Geometry check sheet. Reference: the model listing, model coordinates, mm. A direction names the side the tool comes from. Coordinates: 2 decimals unless noted, no trailing zeros. Write each loop counter-clockwise with the first axis right and the second up, starting at its lowest first coordinate (ties: lowest second). Pieces come first, ordered by that corner, then holes. Notation, with made-up numbers: (-1.75, 63) -> (14.25, 63) arc R9 cw to (14.25, 67) -> close; hole circle Ø10 at (49, 89.25). An arc over 180 degrees is marked (long way). Answer in a Markdown table with one row per item. Add a question column.
Q1. Tool access check on faces 4 (the face through (-65, 60, -62)), 5 (the face through (-173.206, 54.768, -26.385)). Record the directions out of +Z, -Z, +X, -X, +Y, -Y that give a thin tool (end or side, any length) a straight path to the whole face; none if there is none.
Q2. Thickness scan on line 1 (X direction, y = 57.5, z = -85); line 2 (Y direction, x = -34, z = -34.5); line 3 (Y direction, x = 166.5, z = 21). Record the ranges inside material, lowest first.
Q3. Section check D-D, the plane z = 17.5. Record the boundary of the cut face in (x, y), and give its area (3 significant figures).
Q4. Section check A-A, the plane x = -44. Record the boundary of the cut face in (y, z).
Q5. Gauge pin test, flat ends, axial feed: P1, Ø3, axis at x = -179, z = 34.5, coming from the +Y side; P2, Ø4, axis at x = -185.5, z = -23, coming from the +Y side. Record the tip position at first contact, or that the pin passes through.
Q6. Release check for a two-part mould opening along Z. For faces 1 (the face through (-35, 53.5, -24)), 2 (the face through (-9, 30, -108.456)), 3 (the face through (-255.515, 30, -22)) record: pulls with the +Z half, pulls with the -Z half, needs draft (parallel to the pull), parting line crosses it, or undercut.
Q7. Section check B-B, the plane z = 37. Record the boundary of the cut face in (x, y), and give its area (3 significant figures).
Q8. Section check C-C, the plane x = 44. Record the boundary of the cut face in (y, z), and give its area (3 significant figures).
```python
from build123d import *

# Parameters (mm, degrees)
SKETCH1_W           = 500
SKETCH1_H           = 170
BOSS_EXTRUDE1_DEPTH = 60
SKETCH3_R           = 67.5
CUT_EXTRUDE1_DEPTH  = 4
SKETCH4_R           = 25
SKETCH4_R_2         = 22.5
CUT_EXTRUDE2_DEPTH  = 2.5


with BuildPart() as part:
    # Sketch1 → Boss-Extrude1 (new body)
    with BuildSketch(Plane(origin=(0, 0, 0), x_dir=(1, 0, 0), z_dir=(0, 1, 0))):
        with Locations((-5.514705882, 23.455882353)):
            Rectangle(SKETCH1_W, SKETCH1_H)
    extrude(amount=BOSS_EXTRUDE1_DEPTH)

    # Sketch3 → Cut-Extrude1 (cut)
    with BuildSketch(Plane(origin=(0, 60, 0), x_dir=(1, 0, 0), z_dir=(0, 1, 0))):
        with Locations(Location((-5.514705882, 26.094123359, 0), (0, 0, 270))):
            Circle(SKETCH3_R)
        with Locations(Location((154.485294118, 26.094123359, 0), (0, 0, 270))):
            Circle(SKETCH3_R)
        with Locations(Location((-165.514705882, 26.094123359, 0), (0, 0, 270))):
            Circle(SKETCH3_R)
    extrude(amount=-CUT_EXTRUDE1_DEPTH, mode=Mode.SUBTRACT)

    # Sketch4 → Cut-Extrude2 (cut)
    with BuildSketch(Plane(origin=(0, 56, 0), x_dir=(1, 0, 0), z_dir=(0, 1, 0))):
        with Locations(Location((-135.514705882, 23.455882353, 0), (0, 0, 270))):
            Circle(SKETCH4_R)
        with Locations(Location((-195.514705882, 23.455882353, 0), (0, 0, 270))):
            Circle(SKETCH4_R_2)
        with Locations(Location((-35.514705882, 23.455882353, 0), (0, 0, 270))):
            Circle(SKETCH4_R_2)
        with Locations(Location((24.485294118, 23.455882353, 0), (0, 0, 270))):
            Circle(SKETCH4_R)
        with Locations(Location((124.485294118, 23.455882353, 0), (0, 0, 270))):
            Circle(SKETCH4_R_2)
        with Locations(Location((184.485294118, 23.455882353, 0), (0, 0, 270))):
            Circle(SKETCH4_R)
    extrude(amount=-CUT_EXTRUDE2_DEPTH, mode=Mode.SUBTRACT)


solid = part.part
```
Calculated:
| question | item | result |
|---|---|---|
| 1 | face 4 | +Z, -Z, +X, -X, +Y |
| 1 | face 5 | +Y |
| 2 | line 1 | x = -255.51 to -198.47, -132.55 to -38.47, 27.45 to 121.53, 187.45 to 244.49 |
| 2 | line 2 | y = 0 to 53.5 |
| 2 | line 3 | y = 0 to 56 |
| 3 | outline | (-255.51, 0) -> (244.49, 0) -> (244.49, 60) -> (206.02, 60) -> (206.02, 56) -> (102.95, 56) -> (102.95, 60) -> (46.02, 60) -> (46.02, 56) -> (-57.05, 56) -> (-57.05, 60) -> (-113.98, 60) -> (-113.98, 56) -> (-217.05, 56) -> (-217.05, 60) -> (-255.51, 60) -> close |
| 3 | area | 28,800 mm² |
| 4 | outline | (0, -108.46) -> (60, -108.46) -> (60, -81.55) -> (56, -81.55) -> (56, -44.29) -> (53.5, -44.29) -> (53.5, -2.62) -> (56, -2.62) -> (56, 29.36) -> (60, 29.36) -> (60, 61.54) -> (0, 61.54) -> close |
| 5 | P1 | stops at y = 56 |
| 5 | P2 | stops at y = 53.5 |
| 6 | face 1 | undercut |
| 6 | face 2 | pulls with the -Z half |
| 6 | face 3 | needs draft |
| 7 | outline | (-255.51, 0) -> (244.49, 0) -> (244.49, 60) -> (178.47, 60) -> (178.47, 56) -> (130.5, 56) -> (130.5, 60) -> (18.47, 60) -> (18.47, 56) -> (-29.5, 56) -> (-29.5, 60) -> (-141.53, 60) -> (-141.53, 56) -> (-189.5, 56) -> (-189.5, 60) -> (-255.51, 60) -> close |
| 7 | area | 29,400 mm² |
| 8 | outline | (0, -108.46) -> (60, -108.46) -> (60, -71.97) -> (56, -71.97) -> (56, -39.08) -> (53.5, -39.08) -> (53.5, -7.83) -> (56, -7.83) -> (56, 19.78) -> (60, 19.78) -> (60, 61.54) -> (0, 61.54) -> close |
| 8 | area | 9,750 mm² |
